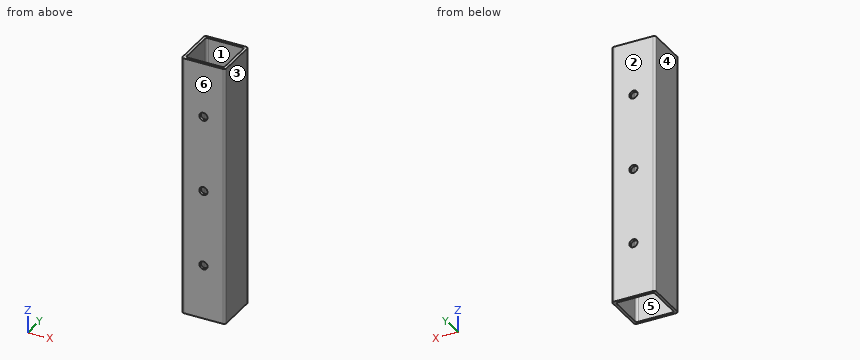
```python
from build123d import *

# Parameters (mm, degrees)
BOSS_EXTRUDE1_DEPTH = 152.4
SKETCH2_R           = 4.7625
CUT_EXTRUDE1_DEPTH  = 76.2


with BuildPart() as part:
    # Sketch1 → Boss-Extrude1 (new, symmetric)
    with BuildSketch(Plane.XY):
        with BuildLine():
            Line((-22.86, -25.4), (22.86, -25.4))
            ThreePointArc((22.86, -25.4), (24.656051224, -24.656051224), (25.4, -22.86))
            Line((25.4, -22.86), (25.4, 22.86))
            ThreePointArc((25.4, 22.86), (24.656051224, 24.656051224), (22.86, 25.4))
            Line((22.86, 25.4), (-22.86, 25.4))
            ThreePointArc((-22.86, 25.4), (-24.656051224, 24.656051224), (-25.4, 22.86))
            Line((-25.4, 22.86), (-25.4, -22.86))
            ThreePointArc((-25.4, -22.86), (-24.656051224, -24.656051224), (-22.86, -25.4))
        make_face()
        with BuildLine():
            Line((-19.685, 22.225), (19.685, 22.225))
            ThreePointArc((19.685, 22.225), (21.481051224, 21.481051224), (22.225, 19.685))
            Line((22.225, 19.685), (22.225, -19.685))
            ThreePointArc((22.225, -19.685), (21.481051224, -21.481051224), (19.685, -22.225))
            Line((19.685, -22.225), (-19.685, -22.225))
            ThreePointArc((-19.685, -22.225), (-21.481051224, -21.481051224), (-22.225, -19.685))
            Line((-22.225, -19.685), (-22.225, 19.685))
            ThreePointArc((-22.225, 19.685), (-21.481051224, 21.481051224), (-19.685, 22.225))
        make_face(mode=Mode.SUBTRACT)
    extrude(amount=BOSS_EXTRUDE1_DEPTH, both=True)

    # Sketch2 → Cut-Extrude1 (cut, symmetric)
    with BuildSketch(Plane(origin=(0, 0, 0), x_dir=(1, 0, 0), z_dir=(0, 1, 0))):
        with Locations(Location((0, 0, 0), (0, 0, 270))):
            Circle(SKETCH2_R)
        with Locations(Location((0, 88.9, 0), (0, 0, 270))):
            Circle(SKETCH2_R)
        with Locations(Location((0, -88.9, 0), (0, 0, 270))):
            Circle(SKETCH2_R)
    extrude(amount=CUT_EXTRUDE1_DEPTH, both=True, mode=Mode.SUBTRACT)


solid = part.part
```
Model file for the job. Use its own axes, mm. Face numbers are marked on the shaded views. A direction names the side the tool comes from. Give positions to 0.01 mm unless a question says otherwise; leave off trailing zeros. Loops run counter-clockwise (first coordinate to the right, second up) from the corner with the lowest first, then second, coordinate; pieces in that order, holes last. Notation, with made-up numbers: (12.5, 39.25) - (69.5, 39.25) arc R14 ccw to (69.5, 50.25) - close; hole circle Ø1 at (76.5, 72). An arc over 180 degrees is marked (long way). One line per item, written item: value. Start each with the question number.
1. Slice it at B-B (z = -29). List the corners of the cut face in (x, y) (3 decimals).
2. Pull direction X, two halves, no side cores. Call the marked faces 3, 4, 5 and 6: pulls with the +X half, pulls with the -X half, needs draft (parallel to the pull), parting line crosses it, or undercut.
3. Which spindle directions (+Z, -Z, +X, -X, +Y, -Y) get a long thin tool onto all of the face, cutting with end or side? Do the marked faces 1 and 2. Say none if no direction does.
4. Slice it at C-C (y = 4). List the corners of the cut face in (x, z) (3 decimals).
5. Slice it at D-D (z = -88.9). List the corners of the cut face in (x, y) (1 decimal), plus the area to 3 significant figures.
6. Slice it at A-A (x = 0). Give the number of separate pieces and of enclosed holes in the cut face, plus the area to 3 significant figures.
7. Probe L1, parallel to X at y = 4, z = -59 (3 decimals); L2, parallel to X at y = 23.2, z = 88.9. List the from-to ranges inside material, lowest first. Write a range as from..to.
Solution:
1. outline: (-25.4, -22.86) arc R2.54 ccw to (-22.86, -25.4) - (22.86, -25.4) arc R2.54 ccw to (25.4, -22.86) - (25.4, 22.86) arc R2.54 ccw to (22.86, 25.4) - (-22.86, 25.4) arc R2.54 ccw to (-25.4, 22.86) - close; hole (-22.225, -19.685) arc R2.54 ccw to (-19.685, -22.225) - (19.685, -22.225) arc R2.54 ccw to (22.225, -19.685) - (22.225, 19.685) arc R2.54 ccw to (19.685, 22.225) - (-19.685, 22.225) arc R2.54 ccw to (-22.225, 19.685) - close
2. face 3: pulls with the +X half
2. face 4: pulls with the -X half
2. face 5: undercut
2. face 6: needs draft
3. face 1: +Z, -Z
3. face 2: +Z, -Z, +X, -X, +Y
4. outline: (-25.4, -152.4) - (-22.225, -152.4) - (-22.225, 152.4) - (-25.4, 152.4) - close; (22.225, -152.4) - (25.4, -152.4) - (25.4, 152.4) - (22.225, 152.4) - close
5. outline: (-25.4, -22.9) arc R2.5 ccw to (-22.9, -25.4) - (-4.8, -25.4) - (-4.8, -22.2) - (-19.7, -22.2) arc R2.5 cw to (-22.2, -19.7) - (-22.2, 19.7) arc R2.5 cw to (-19.7, 22.2) - (-4.8, 22.2) - (-4.8, 25.4) - (-22.9, 25.4) arc R2.5 ccw to (-25.4, 22.9) - close; (4.8, -25.4) - (22.9, -25.4) arc R2.5 ccw to (25.4, -22.9) - (25.4, 22.9) arc R2.5 ccw to (22.9, 25.4) - (4.8, 25.4) - (4.8, 22.2) - (19.7, 22.2) arc R2.5 cw to (22.2, 19.7) - (22.2, -19.7) arc R2.5 cw to (19.7, -22.2) - (4.8, -22.2) - close
5. area: 544 mm^2
6. separate pieces: 8
6. enclosed holes: 0
6. area: 1,750 mm^2
7. L1: x = -25.4..-22.225, 22.225..25.4
7. L2: x = -25.38..-4.76, 4.76..25.38
